The listing builds one solid part. Answer for the finished solid, in the listing's coordinates (mm). Face numbers are marked on the shaded views. A direction names the side the tool comes from. Give positions to 0.01 mm unless a question says otherwise; leave off trailing zeros. Write each loop counter-clockwise with the first axis right and the second up, starting at its lowest first coordinate (ties: lowest second). Pieces come first, ordered by that corner, then holes. Notation, with made-up numbers: (61, -24) -> (93, -24) arc R32 cw to (93, 6) -> close; hole circle Ø4 at (-32, 58.5). An arc over 180 degrees is marked (long way). One line per question, with ' | ' between items.
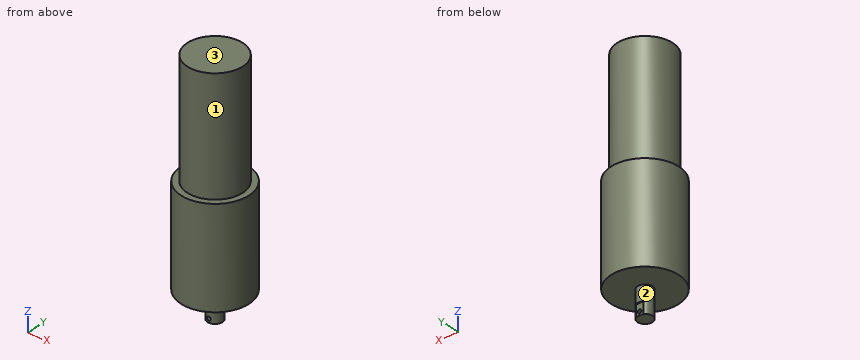
from build123d import *

# Parameters (mm, degrees)
SKETCH1_R           = 18.415
BOSS_EXTRUDE1_DEPTH = 76.2
SKETCH2_R           = 22.54885
BOSS_EXTRUDE2_DEPTH = 65.4177
SKETCH3_R           = 4.9911
BOSS_EXTRUDE3_DEPTH = 17.78
SKETCH5_W           = 5.08
SKETCH5_H           = 1.253731976
CUT_EXTRUDE1_DEPTH  = 7.62
CUT_EXTRUDE2_REACH  = 28.845
SKETCH6_R           = 1.27


with BuildPart() as part:
    # Sketch1 → Boss-Extrude1 (new body)
    with BuildSketch(Plane.XY):
        Circle(SKETCH1_R)
    extrude(amount=BOSS_EXTRUDE1_DEPTH)

    # Sketch2 → Boss-Extrude2 (add)
    with BuildSketch(Plane(origin=(0, 0, 0), x_dir=(-1, 0, 0), z_dir=(0, 0, -1))):
        Circle(SKETCH2_R)
    extrude(amount=BOSS_EXTRUDE2_DEPTH)

    # Sketch3 → Boss-Extrude3 (add)
    with BuildSketch(Plane(origin=(0, 0, -65.4177), x_dir=(-1, 0, 0), z_dir=(0, 0, -1))):
        Circle(SKETCH3_R)
    extrude(amount=BOSS_EXTRUDE3_DEPTH)

    # Sketch5 → Cut-Extrude1 (cut)
    with BuildSketch(Plane(origin=(0, 0, -83.1977), x_dir=(-1, 0, 0), z_dir=(0, 0, -1))):
        with Locations((0, 4.923315593)):
            Rectangle(SKETCH5_W, SKETCH5_H)
    extrude(amount=-CUT_EXTRUDE1_DEPTH, mode=Mode.SUBTRACT)

    # Sketch6 → Cut-Extrude2 (cut, up to next)
    with BuildSketch(Plane(origin=(0, 4.296449605, 0), x_dir=(1, 0, 0), z_dir=(0, 1, 0)), mode=Mode.PRIVATE) as cut_extrude2_sk1:
        with Locations((0, 80.6577)):
            Circle(SKETCH6_R)
    cut_extrude2_tool1 = extrude(cut_extrude2_sk1.sketch, amount=-CUT_EXTRUDE2_REACH, mode=Mode.PRIVATE) & part.part
    add(cut_extrude2_tool1.solids().sort_by_distance((0, 4.29645, -80.6577))[0], mode=Mode.SUBTRACT)


solid = part.part
Item 1: Flat-ended cylindrical pins translate along their axes: pin 1 (1 mm diameter, centred on x = -2.5, z = -39.5, fed in from +Y); pin 2 (3 mm diameter, centred on y = 14, z = -48.5, fed in from -X); pin 3 (5 mm diameter, centred on x = 10.5, z = -61, fed in from +Y). Find the tip coordinate at first contact, or state that the pin passes through.
Answers below:
pin 1: y = 22.46 | pin 2: x = -18.77 | pin 3: y = 21.08
Item 2: Find section A-A (y = -12.5). Write down the section's boundary in (x, z).
Answers below:
outline: (-18.77, -65.42) -> (18.77, -65.42) -> (18.77, 0) -> (13.52, 0) -> (13.52, 76.2) -> (-13.52, 76.2) -> (-13.52, 0) -> (-18.77, 0) -> close
Item 3: Find section C-C (z = 21). Write down the section's boundary in (x, y) (3 decimals).
Answers below:
outline: circle Ø36.83 at (0, 0)
Item 4: A tool of negligible diameter and unlimited length cuts with its end or side. For the marked faces 1, 2 and 3, from which of +Z, -Z, +X, -X, +Y, -Y can it reach the whole face along a straight path? Write none if from no direction.
Answers below:
face 1: +Z | face 2: -Z | face 3: +Z, +X, -X, +Y, -Y
Item 5: Find section D-D (y = 0). Write down the section's boundary in (x, z) (3 decimals).
Answers below:
outline: (-22.549, -65.418) -> (-4.991, -65.418) -> (-4.991, -83.198) -> (4.991, -83.198) -> (4.991, -65.418) -> (22.549, -65.418) -> (22.549, 0) -> (18.415, 0) -> (18.415, 76.2) -> (-18.415, 76.2) -> (-18.415, 0) -> (-22.549, 0) -> close; hole circle Ø2.54 at (0, -80.658)
Item 6: Find section B-B (x = -15). Write down the section's boundary in (y, z).
Answers below:
outline: (-16.84, -65.42) -> (16.84, -65.42) -> (16.84, 0) -> (10.68, 0) -> (10.68, 76.2) -> (-10.68, 76.2) -> (-10.68, 0) -> (-16.84, 0) -> close
Item 7: Consider line 1 (Z direction, x = 0, y = 0.75); line 2 (Z direction, x = -16, y = -7.5); line 3 (Y direction, x = -19, z = -56.5). Determine where each line is inside the solid, lowest interval first. Write a range as [from, to].
Answers below:
line 1: [-83.2, -81.93], [-79.39, 76.2] | line 2: [-65.42, 76.2] | line 3: [-12.14, 12.14]
